Part model, mm, in its own coordinate system. Coordinates: 2 decimals unless noted, no trailing zeros. Loops run counter-clockwise (first coordinate to the right, second up) from the corner with the lowest first, then second, coordinate; pieces in that order, holes last. Notation, with made-up numbers: (38, -14) -> (83, -14) arc R27 ccw to (83, 23) -> close; hole circle Ø2 at (73, -28). An arc over 180 degrees is marked (long way). Use one line per item in the form item = value. Start each with the question number.
(1) Drill centre lines: L1, parallel to Y at x = 2.5, z = 6 (3 decimals); L2, parallel to Z at x = 4.75, y = 0 (3 decimals); L3, parallel to Y at x = 0, z = 8. Where is each one in solid material? Low to high. Write a range as [from, to].
(2) Pin check, flat tips, straight feed: P1, Ø4, axis at y = 0, z = 6, coming from the +X side; P2, Ø1, axis at x = 8, y = -4, coming from the +Z side; P3, Ø5.5, axis at x = 0, y = 0, coming from the -Z side (3 decimals). Stop position of each tip, or through.
(3) Band-saw the part on D-D on z = 2.5. Give the cut face in (x, y).
(4) Band-saw the part on A-A on y = 0. Give the cut face in (x, z) (3 decimals).
(5) Mould opens along Z. For faces 1 (the flat face through (4, 0, 12)), 2 (the flat face through (4, 0, 0)), 3 (the cylindrical face through (6.18, 2.93, 4.78)), 4 (the flat face through (10, 3, 3)) say: +Z half, -Z half, draft (parallel to the pull), parting line (faces both ways), or undercut.
(6) Band-saw the part on C-C on x = 0.75. Give the cut face in (y, z) (3 decimals).
(7) Band-saw the part on B-B on x = 8.5. Give the cut face in (y, z) (3 decimals), then the cut area to 3 significant figures.
```python
from build123d import *

# Parameters (mm, degrees)
SKETCH1_W           = 15
SKETCH1_H           = 12
SKETCH1_R           = 3
BOSS_EXTRUDE1_DEPTH = 12
SKETCH2_R           = 3.175
CUT_EXTRUDE1_DEPTH  = 10
FILLET1_R           = 3


with BuildPart() as part:
    # Sketch1 → Boss-Extrude1 (new body)
    with BuildSketch(Plane.XY):
        with Locations((2.5, 0)):
            Rectangle(SKETCH1_W, SKETCH1_H)
        Circle(SKETCH1_R, mode=Mode.SUBTRACT)
    extrude(amount=BOSS_EXTRUDE1_DEPTH)

    # Sketch2 → Cut-Extrude1 (cut)
    with BuildSketch(Plane(origin=(10, 0, 0), x_dir=(0, 0, -1), z_dir=(1, 0, 0))):
        with Locations(Location((-6, 0, 0), (0, 0, 90))):
            Circle(SKETCH2_R)
    extrude(amount=-CUT_EXTRUDE1_DEPTH, mode=Mode.SUBTRACT)

    # Fillet1
    fillet1_edges = [part.edges().sort_by_distance(p)[0] for p in [
        (2.5, 6, 12),
        (2.5, 6, 0),
        (2.5, -6, 0),
        (2.5, -6, 12),
    ]]
    fillet(fillet1_edges, radius=FILLET1_R - 0.0001)  # a hair under: the kernel refuses the full size


solid = part.part
```
A:
q1.L1 = [-6, -3.175], [3.175, 6]
q1.L2 = [0, 2.825], [9.175, 12]
q1.L3 = [-6, -3], [3, 6]
q2.P1 = -2.24
q2.P2 = 11.96
q2.P3 = through
q3.outline = (-5, -5.96) -> (10, -5.96) -> (10, 5.96) -> (-5, 5.96) -> close; hole circle Ø6 at (0, 0)
q4.outline = (-5, 0) -> (-3, 0) -> (-3, 12) -> (-5, 12) -> close; (3, 0) -> (10, 0) -> (10, 2.825) -> (3, 2.825) -> close; (3, 9.175) -> (10, 9.175) -> (10, 12) -> (3, 12) -> close
q5.face_1 = +Z half
q5.face_2 = -Z half
q5.face_3 = undercut
q5.face_4 = draft
q6.outline = (-6, 3) arc R3 ccw to (-3, 0) -> (-2.905, 0) -> (-2.905, 4.718) arc R3.175 cw to (-2.905, 7.282) -> (-2.905, 12) -> (-3, 12) arc R3 ccw to (-6, 9) -> close; (2.905, 0) -> (3, 0) arc R3 ccw to (6, 3) -> (6, 9) arc R3 ccw to (3, 12) -> (2.905, 12) -> (2.905, 7.282) arc R3.175 cw to (2.905, 4.718) -> close
q7.outline = (-6, 3) arc R3 ccw to (-3, 0) -> (3, 0) arc R3 ccw to (6, 3) -> (6, 9) arc R3 ccw to (3, 12) -> (-3, 12) arc R3 ccw to (-6, 9) -> close; hole circle Ø6.35 at (0, 6)
q7.area = 105 mm²
